Build history of the part. All positions in model axes, mm. Coordinates: 2 decimals unless noted, no trailing zeros.
Item 1: Drill centre lines: line 1 along X through (y, z) = (8.5, 0.9); line 2 along X through (y, z) = (10.75, 0.75); line 3 along Y through (x, z) = (1, 1.45). Where is each one in solid material? Low to high.
Item 2: Mould opens along X. For faces 1 (the face through (-3.51, -11.83, 1.57)), 2 (the face through (-10.822, 5.878, 1.565)) say: released by +X, released by -X, zero draft, split by the parting line, or undercut.
Item 3: Flat gauge pin, fed straight in: pin 1 (1.5 mm diameter, centred on y = -9.5, z = 0.5, fed in from -X). Where does the tip first touch, or does it go through?
from build123d import *

# Parameters (mm, degrees)
F2_DEPTH = 3.175
F3_D     = 3.175


with BuildPart() as f2:
    # F1 (on Top) → F2 (new body)
    with BuildSketch(Plane.XY):
        Polygon((0.65056, 13.217399), (0, 11.43), (-0.65056, 13.217399), (-1.080222, 13.189238), (-1.491914, 11.332215), (-2.370211, 13.019408), (-2.792522, 12.935405), (-2.958302, 11.040532), (-4.049308, 12.59865), (-4.457041, 12.460243), (-4.374072, 10.559943), (-5.659119, 11.962326), (-6.045298, 11.771884), (-5.715, 9.89867), (-7.172101, 11.121324), (-7.530119, 10.882104), (-6.958143, 9.068029), (-8.562367, 10.090032), (-8.886097, 9.806128), (-8.082231, 8.082231), (-9.806128, 8.886097), (-10.090032, 8.562367), (-9.068029, 6.958143), (-10.882104, 7.530119), (-11.121324, 7.172101), (-9.89867, 5.715), (-11.771884, 6.045298), (-11.962326, 5.659119), (-10.559943, 4.374072), (-12.460243, 4.457041), (-12.59865, 4.049308), (-11.040532, 2.958302), (-12.935405, 2.792522), (-13.019408, 2.370211), (-11.332215, 1.491914), (-13.189238, 1.080222), (-13.217399, 0.65056), (-11.43, 0), (-13.217399, -0.65056), (-13.189238, -1.080222), (-11.332215, -1.491914), (-13.019408, -2.370211), (-12.935405, -2.792522), (-11.040532, -2.958302), (-12.59865, -4.049308), (-12.460243, -4.457041), (-10.559943, -4.374072), (-11.962326, -5.659119), (-11.771884, -6.045298), (-9.89867, -5.715), (-11.121324, -7.172101), (-10.882104, -7.530119), (-9.068029, -6.958143), (-10.090032, -8.562367), (-9.806128, -8.886097), (-8.082231, -8.082231), (-8.886097, -9.806128), (-8.562367, -10.090032), (-6.958143, -9.068029), (-7.530119, -10.882104), (-7.172101, -11.121324), (-5.715, -9.89867), (-6.045298, -11.771884), (-5.659119, -11.962326), (-4.374072, -10.559943), (-4.457041, -12.460243), (-4.049308, -12.59865), (-2.958302, -11.040532), (-2.792522, -12.935405), (-2.370211, -13.019408), (-1.491914, -11.332215), (-1.080222, -13.189238), (-0.65056, -13.217399), (0, -11.43), (0.65056, -13.217399), (1.080222, -13.189238), (1.491914, -11.332215), (2.370211, -13.019408), (2.792522, -12.935405), (2.958302, -11.040532), (4.049308, -12.59865), (4.457041, -12.460243), (4.374072, -10.559943), (5.659119, -11.962326), (6.045298, -11.771884), (5.715, -9.89867), (7.172101, -11.121324), (7.530119, -10.882104), (6.958143, -9.068029), (8.562367, -10.090032), (8.886097, -9.806128), (8.082231, -8.082231), (9.806128, -8.886097), (10.090032, -8.562367), (9.068029, -6.958143), (10.882104, -7.530119), (11.121324, -7.172101), (9.89867, -5.715), (11.771884, -6.045298), (11.962326, -5.659119), (10.559943, -4.374072), (12.460243, -4.457041), (12.59865, -4.049308), (11.040532, -2.958302), (12.935405, -2.792522), (13.019408, -2.370211), (11.332215, -1.491914), (13.189238, -1.080222), (13.217399, -0.65056), (11.43, 0), (13.217399, 0.65056), (13.189238, 1.080222), (11.332215, 1.491914), (13.019408, 2.370211), (12.935405, 2.792522), (11.040532, 2.958302), (12.59865, 4.049308), (12.460243, 4.457041), (10.559943, 4.374072), (11.962326, 5.659119), (11.771884, 6.045298), (9.89867, 5.715), (11.121324, 7.172101), (10.882104, 7.530119), (9.068029, 6.958143), (10.090032, 8.562367), (9.806128, 8.886097), (8.082231, 8.082231), (8.886097, 9.806128), (8.562367, 10.090032), (6.958143, 9.068029), (7.530119, 10.882104), (7.172101, 11.121324), (5.715, 9.89867), (6.045298, 11.771884), (5.659119, 11.962326), (4.374072, 10.559943), (4.457041, 12.460243), (4.049308, 12.59865), (2.958302, 11.040532), (2.792522, 12.935405), (2.370211, 13.019408), (1.491914, 11.332215), (1.080222, 13.189238), align=None)
    extrude(amount=F2_DEPTH)

    # F3 (through all)
    with Locations(Plane(origin=(0, 0, 0), x_dir=(1, 0, 0), z_dir=(0, 0, -1))):
        with Locations((0, 0)):
            Hole(F3_D / 2)


solid = f2.part
Filled sheet:
1. line 1: x = -10.05 to -8.98, -8.28 to 8.28, 8.98 to 10.05
1. line 2: x = -7.49 to -6.73, -5.87 to -4.55, -4.38 to 4.38, 4.55 to 5.87, 6.73 to 7.49
1. line 3: y = -13.19 to -1.23, 1.23 to 13.19
2. face 1: undercut
2. face 2: undercut
3. pin 1: stops at x = -9.93
